CAD build for the part. Positions are in the model's coordinates, mm. A direction names the side the tool comes from. Coordinates: 2 decimals unless noted, no trailing zeros. Order: outer loops, then holes, each group sorted by start corner. A loop starts at its lowest first (then second) coordinate and runs counter-clockwise, first axis right, second up. Notation, with made-up numbers: (-10.75, -24.5) - (18.25, -24.5) arc R12 cw to (18.25, -15.5) - close; hole circle Ø8 at (78.25, 20.25). An arc over 180 degrees is marked (long way). Return JSON: item names as keys, results as strings.
from build123d import *

# Parameters (mm, degrees)
SKETCH_1_W          = 34.2
SKETCH_1_H          = 12.6
EXTRUDE_1_DEPTH     = 1
SKETCH_2_R          = 2.5
EXTRUDE_2_DEPTH     = 6
SKETCH_3_R          = 1.5
EXTRUDE_3_DEPTH     = 5.5
DOME_3_FACE_RADIUS  = 1.5
DOME_3_HEIGHT       = 0.5
SKETCH_4_R          = 1.5
CUT_EXTRUDE_1_DEPTH = 20.185932346
EXTRUDE_START       = 2
SKETCH_5_R          = 3
SKETCH_5_R_2        = 1.5
EXTRUDE_4_DEPTH     = 2
SKETCH_6_W          = 4.5
SKETCH_6_H          = 8
EXTRUDE_6_DEPTH     = 6
SKETCH_7_W          = 3.38323666
SKETCH_7_H          = 6.498483094
CUT_EXTRUDE_2_DEPTH = 5


with BuildPart() as part:
    # 草图1 → 凸台-拉伸1 (new body)
    with BuildSketch(Plane(origin=(0, 0, 0), x_dir=(1, 0, 0), z_dir=(0, 1, 0))):
        Rectangle(SKETCH_1_W, SKETCH_1_H)
    extrude(amount=EXTRUDE_1_DEPTH)

    # 草图2 → 凸台-拉伸2 (add)
    with BuildSketch(Plane(origin=(0, 1, 0), x_dir=(1, 0, 0), z_dir=(0, 1, 0))):
        with Locations(Location((-12.1, 0, 0), (0, 0, 270))):
            Circle(SKETCH_2_R)
    extrude(amount=EXTRUDE_2_DEPTH)

    # 草图3 → 凸台-拉伸3 (add)
    with BuildSketch(Plane(origin=(0, 1, 0), x_dir=(1, 0, 0), z_dir=(0, 1, 0))):
        with Locations(Location((-6.786156124, 0, 0), (0, 0, 270))):
            Circle(SKETCH_3_R)
    extrude(amount=EXTRUDE_3_DEPTH)

    # 圆顶3: a dome of height H over a round flat face of radius A is a cap of a sphere of radius (A * A + H * H) / (2 * H)
    dome_3_r = (DOME_3_FACE_RADIUS * DOME_3_FACE_RADIUS + DOME_3_HEIGHT * DOME_3_HEIGHT) / (2 * DOME_3_HEIGHT)
    dome_3_base = Plane((-6.786156124, 6.5, 0), z_dir=(0, 1, 0))
    with Locations(dome_3_base.offset(DOME_3_HEIGHT - dome_3_r)):
        dome_3_ball = Sphere(dome_3_r, mode=Mode.PRIVATE)
    add(split(dome_3_ball, bisect_by=dome_3_base, keep=Keep.TOP, mode=Mode.PRIVATE))

    # 草图4 → 切除-拉伸1 (cut, through all)
    with BuildSketch(Plane(origin=(0, 1, 0), x_dir=(1, 0, 0), z_dir=(0, 1, 0))):
        with Locations(Location((7.02445794, 0, 0), (0, 0, 270))):
            Circle(SKETCH_4_R)
    extrude(amount=-CUT_EXTRUDE_1_DEPTH, mode=Mode.SUBTRACT)

    # 草图5 → 凸台-拉伸4 (add)
    with BuildSketch(Plane(origin=(0, 1, 0), x_dir=(1, 0, 0), z_dir=(0, 1, 0)).offset(EXTRUDE_START)):
        with Locations(Location((7.02445794, 0, 0), (0, 0, 270))):
            Circle(SKETCH_5_R)
        with Locations(Location((7.02445794, 0, 0), (0, 0, 270))):
            Circle(SKETCH_5_R_2, mode=Mode.SUBTRACT)
    extrude(amount=-EXTRUDE_4_DEPTH)

    # 草图6 → 凸台-拉伸6 (add)
    with BuildSketch(Plane(origin=(0, 0, 0), x_dir=(-1, 0, 0), z_dir=(0, -1, 0))):
        with Locations((-14.85, 0)):
            Rectangle(SKETCH_6_W, SKETCH_6_H)
    extrude(amount=EXTRUDE_6_DEPTH)

    # 草图7 → 切除-拉伸2 (cut)
    with BuildSketch(Plane.XZ.offset(6)):
        with Locations((14.85, 0)):
            Rectangle(SKETCH_7_W, SKETCH_7_H)
    extrude(amount=-CUT_EXTRUDE_2_DEPTH, mode=Mode.SUBTRACT)


solid = part.part
Item 1: Band-saw the part on A-A, the plane y = -2.5. List the corners of the cut face in (x, z).
Findings below:
{"outline": "(12.6, -4) - (17.1, -4) - (17.1, 4) - (12.6, 4) - close; hole (13.16, -3.25) - (16.54, -3.25) - (16.54, 3.25) - (13.16, 3.25) - close"}
Item 2: Wall check: L1, parallel to X at y = 1.75, z = 0; L2, parallel to Z at x = 14, y = -5; L3, parallel to X at y = 0.7, z = 0. Give the ranges that are in metal, low to high. Write a range as [from, to].
Findings below:
{"L1": "x = [-14.6, -9.6], [-8.29, -5.29], [4.02, 5.52], [8.52, 10.02]", "L2": "z = [-4, -3.25], [3.25, 4]", "L3": "x = [-17.1, 5.52], [8.52, 17.1]"}
Item 3: Band-saw the part on C-C, the plane x = -12.1. List the corners of the cut face in (y, z).
Findings below:
{"outline": "(0, -6.3) - (1, -6.3) - (1, -2.5) - (7, -2.5) - (7, 2.5) - (1, 2.5) - (1, 6.3) - (0, 6.3) - close"}
Item 4: Which spindle directions (+Z, -Z, +X, -X, +Y, -Y) get a long thin tool onto all of the face, cutting with end or side? Do faces 4 (the flat face through (13.158, -4, 0)), 5 (the flat face through (15, -3, 4)), 6 (the cylindrical face through (-8.25, 3.71, -0.33)). Say none if no direction does.
Findings below:
{"face 4": "-Y", "face 5": "+Z, +X, -X, -Y", "face 6": "+Y"}
Item 5: Mould opens along Z. For faces 1 (the flat face through (12.6, -3, 0)), 2 (the flat face through (15, -4, 3.249)), 3 (the flat face through (-0.2, 0.5, 6.3)) say: released by +Z, released by -Z, zero draft, split by the parting line, or undercut.
Findings below:
{"face 1": "zero draft", "face 2": "undercut", "face 3": "released by +Z"}
Item 6: Band-saw the part on D-D, the plane y = 2.5. List the corners of the cut face in (x, z).
Findings below:
{"outline": "circle Ø5 at (-12.1, 0); circle Ø3 at (-6.79, 0); circle Ø6 at (7.02, 0); hole circle Ø3 at (7.02, 0)"}
Item 7: Drop flat-ended pins along their axis: P1, Ø1.7, axis at x = 14.5, y = -4.5, coming from the +Z side; P2, Ø6.5, axis at x = 6, z = 1, coming from the +Y side; P3, Ø2.5, axis at x = 15.5, y = -3.5, coming from the -Z side. Give the stop position or say it passes through.
Findings below:
{"P1": "stops at z = 4", "P2": "stops at y = 3", "P3": "stops at z = -4"}
Item 8: Band-saw the part on B-B, the plane z = 0. List the corners of the cut face in (x, y), then the cut area to 3 significant figures.
Findings below:
{"outline": "(-17.1, 0) - (5.52, 0) - (5.52, 3) - (4.02, 3) - (4.02, 1) - (-5.29, 1) - (-5.29, 6.5) arc R2.5 ccw to (-8.29, 6.5) - (-8.29, 1) - (-9.6, 1) - (-9.6, 7) - (-14.6, 7) - (-14.6, 1) - (-17.1, 1) - close; (8.52, 0) - (12.6, 0) - (12.6, -6) - (13.16, -6) - (13.16, -1) - (16.54, -1) - (16.54, -6) - (17.1, -6) - (17.1, 1) - (10.02, 1) - (10.02, 3) - (8.52, 3) - close", "area": "94.8 mm²"}
